Here's how the part is built. I have some questions about the finished solid (model axes, mm). A direction names the side the tool comes from. Round coordinates to 2 decimals unless told otherwise and drop trailing zeros. Write each loop counter-clockwise with the first axis right and the second up, starting at its lowest first coordinate (ties: lowest second). Pieces come first, ordered by that corner, then holes. Notation, with made-up numbers: (44.25, -35.5) - (57.25, -35.5) arc R28 cw to (57.25, -8.5) - close; hole circle Ø9 at (-34.75, 64). An arc over 180 degrees is marked (long way). One line per item, written item: value. Start each with the question number.
Item 1: For P1, Ø0.9, axis at y = -6, z = -0.5, coming from the +X side; P2, Ø2, axis at x = -5.5, y = -9, coming from the +Z side; P3, Ø0.6, axis at x = -8.5, z = -1.5, coming from the +Y side; P4, Ø2, axis at x = 4, y = 1.5, coming from the -Z side, each with a flat end and sliding along its axis, tell me the tip position at first contact or that it passes through.
Item 2: Imagine slicing it at A-A, the plane y = -5.25. Please give me the cut outline in (x, z).
Item 3: Thinking about a two-plate mould opening in X: for faces 1 (the face through (2, -2, -0.8)), 2 (the face through (5, 0, 4)), 3 (the face through (1.8, 0.1, 1.7)), 4 (the face through (-9, 0, -1)), which applies, released by +X, released by -X, zero draft, split by the parting line, or undercut?
Item 4: If I drill on line 1 (Z direction, x = 1.5, y = -11); line 2 (X direction, y = 2, z = 1.85); line 3 (Z direction, x = -6.25, y = 1.5), over which ranges is the centre line in solid material (lowest first)?
Item 5: Imagine slicing it at B-B, the plane x = -5. Please give me the cut outline in (y, z), then the cut area to 3 significant figures.
Item 6: For faces 5 (the face through (2, -2, 0)), 6 (the face through (9, 0, -1)), which set-ups out of +Z, -Z, +X, -X, +Y, -Y let a thin tool reach every point of the face, with its end or its side?
Item 7: Imagine slicing it at D-D, the plane z = 2.2. Please give me the cut outline in (x, y), then the cut area to 3 significant figures.
Item 8: Imagine slicing it at C-C, the plane y = 0. Please give me the cut outline in (x, z), then the cut area to 3 significant figures.
```python
from build123d import *

# Parameters (mm, degrees)
SKETCH_2_R        = 3.2
EXTRUDE_1_DEPTH   = 4
EXTRUDE_1_2_DEPTH = 4
SKETCH_3_W        = 8
SKETCH_3_H        = 8
EXTRUDE_2_DEPTH   = 0.8
SKETCH_4_W        = 2
SKETCH_4_H        = 2
EXTRUDE_3_DEPTH   = 0.8
SKETCH_5_W        = 6
SKETCH_5_H        = 1.2
SKETCH_5_W_2      = 1.2
SKETCH_5_H_2      = 8
EXTRUDE_4_DEPTH   = 0.8
FILLET_1_R        = 0.5


with BuildPart() as part:
    # Sketch 2 → Extrude 1 (new body)
    with BuildSketch(Plane.XY):
        with Locations((-5, 0)):
            Circle(SKETCH_2_R)
    extrude(amount=EXTRUDE_1_DEPTH)



with BuildPart() as body_2:
    # Sketch 2 → Extrude 1 2 (new body)
    with BuildSketch(Plane.XY):
        with Locations((5, 0)):
            Circle(SKETCH_2_R)
    extrude(amount=EXTRUDE_1_2_DEPTH)


with BuildPart() as part_1:
    add(part.part)

    add(body_2.part)  # Extrude 2 merges body 2
    # Sketch 3 → Extrude 2 (add)
    with BuildSketch(Plane(origin=(0, 0, 0), x_dir=(-1, 0, 0), z_dir=(0, 0, -1))):
        with Locations((-5, 0)):
            Rectangle(SKETCH_3_W, SKETCH_3_H)
        with Locations((5, 0)):
            Rectangle(SKETCH_3_W, SKETCH_3_H)
    extrude(amount=EXTRUDE_2_DEPTH)

    # Sketch 4 → Extrude 3 (add)
    with BuildSketch(Plane(origin=(0, 0, -0.8), x_dir=(-1, 0, 0), z_dir=(0, 0, -1))):
        with Locations((-8, 0.7)):
            Rectangle(SKETCH_4_W, SKETCH_4_H)
        with Locations((8, 0.7)):
            Rectangle(SKETCH_4_W, SKETCH_4_H)
    extrude(amount=EXTRUDE_3_DEPTH)

    # Sketch 5 → Extrude 4 (add)
    with BuildSketch(Plane(origin=(0, 0, -0.8), x_dir=(-1, 0, 0), z_dir=(0, 0, -1))):
        Polygon((-3, -10.8), (-3, -4), (-4.2, -4), (-4.2, -12), (-3, -12), align=None)
        with Locations((0, -11.4)):
            Rectangle(SKETCH_5_W, SKETCH_5_H)
        with Locations((3.6, -8)):
            Rectangle(SKETCH_5_W_2, SKETCH_5_H_2)
    extrude(amount=-EXTRUDE_4_DEPTH)

    # Fillet 1
    fillet_1_edges = [part_1.edges().sort_by_distance(p)[0] for p in [
        (-8.2, 0, 4),
        (1.8, 0, 4),
    ]]
    fillet(fillet_1_edges, radius=FILLET_1_R)


solid = part_1.part
```
Values follow:
1. P1: stops at x = 4.2
1. P2: passes through
1. P3: stops at y = 1.7
1. P4: stops at z = -0.8
2. outline: (-4.2, -0.8) - (-3, -0.8) - (-3, 0) - (-4.2, 0) - close; (3, -0.8) - (4.2, -0.8) - (4.2, 0) - (3, 0) - close
3. face 1: undercut
3. face 2: zero draft
3. face 3: undercut
3. face 4: released by -X
4. line 1: z = -0.8 to 0
4. line 2: x = -7.5 to -2.5, 2.5 to 7.5
4. line 3: z = -0.8 to 4
5. outline: (-4, -0.8) - (4, -0.8) - (4, 0) - (3.2, 0) - (3.2, 3.5) arc R0.5 ccw to (2.7, 4) - (-2.7, 4) arc R0.5 ccw to (-3.2, 3.5) - (-3.2, 0) - (-4, 0) - close
5. area: 31.9 mm^2
6. face 5: +Z
6. face 6: +Z, -Z, +X, +Y, -Y
7. outline: circle Ø6.4 at (-5, 0); circle Ø6.4 at (5, 0)
7. area: 64.3 mm^2
8. outline: (-9, -1.6) - (-7, -1.6) - (-7, -0.8) - (-1, -0.8) - (-1, 0) - (-1.8, 0) - (-1.8, 3.5) arc R0.5 ccw to (-2.3, 4) - (-7.7, 4) arc R0.5 ccw to (-8.2, 3.5) - (-8.2, 0) - (-9, 0) - close; (1, -0.8) - (7, -0.8) - (7, -1.6) - (9, -1.6) - (9, 0) - (8.2, 0) - (8.2, 3.5) arc R0.5 ccw to (7.7, 4) - (2.3, 4) arc R0.5 ccw to (1.8, 3.5) - (1.8, 0) - (1, 0) - close
8. area: 67.0 mm^2
